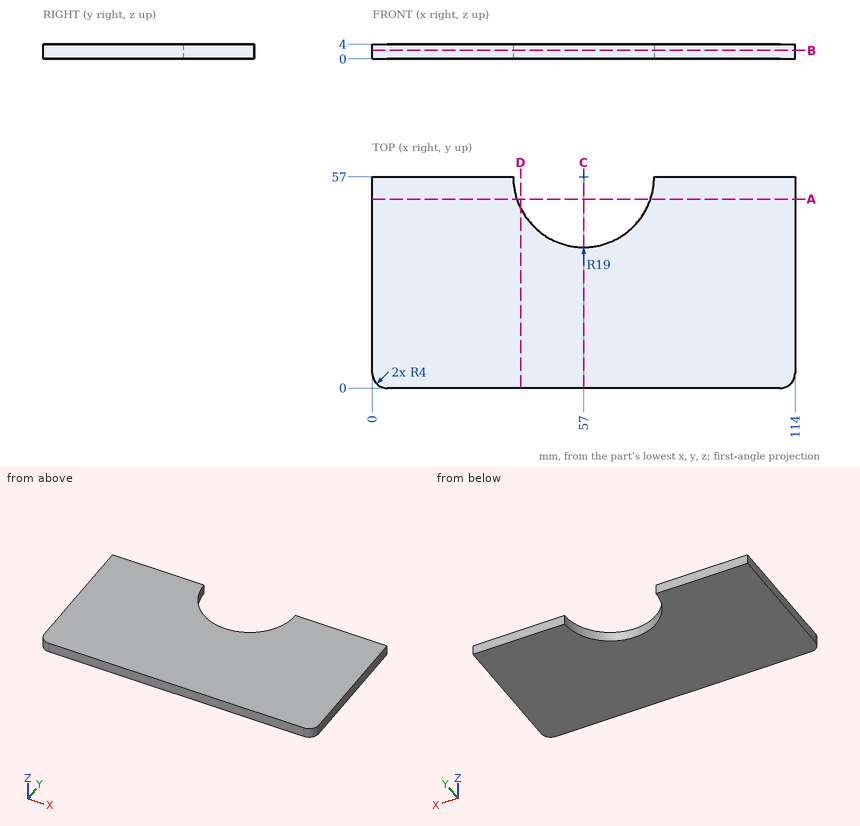
Verification items for this drawing (mm, ordinates from the low corner). Coordinates: 2 decimals unless noted, no trailing zeros. Write each loop counter-clockwise with the first axis right and the second up, starting at its lowest first coordinate (ties: lowest second). Pieces come first, ordered by that corner, then holes. Notation, with made-up numbers: M 42.25,49 L 91.25,49 A26 ccw 91.25,88 Z; hole C -33.75,53 d2. An arc over 180 degrees is marked long. Use one line per item in the form item = value. Start each with the question number.
1) Thickness scan on probe 1 along X at (y, z) = (43, 0.8); probe 2 along X at (y, z) = (53.5, 1.35); probe 3 along Y at (x, z) = (43.5, 1.5). Record the ranges inside material, lowest first. Write a range as from..to.
2) Section check A-A on y = 51. Enter the section's corners in (x, z), and give its area (3 significant figures).
3) Section check B-B on z = 2.3. Enter the section's corners in (x, y), and give its area (3 significant figures).
4) Section check D-D on x = 40. Enter the section's corners in (y, z).
5) Section check C-C on x = 57. Enter the section's corners in (y, z).
6) Go/stop test with flat-tipped pins: pin 1 Ø1.5 at (x, z) = (70, 3.5) entering from +Y; pin 2 Ø1.5 at (x, z) = (48.5, 3) entering from +Y. Record where each tip stops, or that it passes through.
Responses:
q1.probe_1 = 0..44.15, 69.85..114
q1.probe_2 = 0..38.33, 75.67..114
q1.probe_3 = 0..43.63
q2.outline = M 0,0 L 38.97,0 L 38.97,4 L 0,4 Z; M 75.03,0 L 114,0 L 114,4 L 75.03,4 Z
q2.area = 312 mm2
q3.outline = M 0,4 A4 ccw 4,0 L 110,0 A4 ccw 114,4 L 114,57 L 76,57 A19 cw 38,57 L 0,57 Z
q3.area = 5,920 mm2
q4.outline = M 0,0 L 48.51,0 L 48.51,4 L 0,4 Z
q5.outline = M 0,0 L 38,0 L 38,4 L 0,4 Z
q6.pin_1 = 43.89
q6.pin_2 = 40.4
